from build123d import *

# Parameters (mm, degrees)
SKETCH1_W                  = 120
SKETCH1_H                  = 60
BOSS_EXTRUDE1_DEPTH        = 10
BOSS_EXTRUDE2_DEPTH        = 10
F_25_0_28_DIAMETER_HOLE1_D = 28
BOSS_EXTRUDE3_DEPTH        = 5
CUT_EXTRUDE1_DEPTH         = 147.130542204
SKETCH7_R                  = 16
SKETCH7_R_2                = 11.5
BOSS_EXTRUDE4_DEPTH        = 22.5
BOSS_EXTRUDE5_DEPTH        = 16
CUT_EXTRUDE2_START         = -10
CUT_EXTRUDE2_DEPTH         = 20
BOSS_EXTRUDE6_DEPTH        = 14.5
BOSS_EXTRUDE6_DEPTH_BACK   = 22.5
FILLET1_R                  = 2


# Read off the part's stored shape, not the designer's step: Cut-Extrude2
with BuildPart() as part:
    # Sketch1 → Boss-Extrude1 (new body)
    with BuildSketch(Plane(origin=(0, 0, 0), x_dir=(1, 0, 0), z_dir=(0, 1, 0))):
        with Locations((60, 30)):
            Rectangle(SKETCH1_W, SKETCH1_H)
    extrude(amount=BOSS_EXTRUDE1_DEPTH)

    # Sketch2 → Boss-Extrude2 (add)
    with BuildSketch(Plane.XY):
        with BuildLine():
            Line((0, 10), (0, 0))
            Line((0, 0), (70.357344256, -43.964148108))
            ThreePointArc((70.357344256, -43.964148108), (92.522919584, -46.524792309), (108.511026917, -30.960408214))
            Line((108.511026917, -30.960408214), (120, 0))
            Line((120, 0), (120, 10))
            Line((120, 10), (0, 10))
        make_face()
    boss_extrude2 = extrude(amount=-BOSS_EXTRUDE2_DEPTH)

    # Mirror1: Boss-Extrude2 across plane
    add(boss_extrude2.mirror(Plane.XY.offset(-30)))

    # 25.0 _28_ Diameter Hole1 (through all)
    with Locations(Plane(origin=(84.135245127, -21.914897608, 0), x_dir=(1, 0, 0), z_dir=(0, 0, 1))):
        with Locations((0, 0)):
            Hole(F_25_0_28_DIAMETER_HOLE1_D / 2)

    # Sketch5 → Boss-Extrude3 (add)
    with BuildSketch(Plane(origin=(0, 10, 0), x_dir=(1, 0, 0), z_dir=(0, 1, 0))):
        with BuildLine():
            Line((100, 18), (68, 18))
            ThreePointArc((68, 18), (56, 30), (68, 42))
            Line((68, 42), (100, 42))
            ThreePointArc((100, 42), (112, 30), (100, 18))
        make_face()
        with BuildLine():
            Line((100, 24), (68, 24))
            ThreePointArc((68, 24), (62, 30), (68, 36))
            Line((68, 36), (100, 36))
            ThreePointArc((100, 36), (106, 30), (100, 24))
        make_face(mode=Mode.SUBTRACT)
    extrude(amount=BOSS_EXTRUDE3_DEPTH)

    # Sketch5_2 → Cut-Extrude1 (cut, through all)
    with BuildSketch(Plane(origin=(0, 10, 0), x_dir=(1, 0, 0), z_dir=(0, 1, 0))):
        with BuildLine():
            Line((100, 36), (68, 36))
            ThreePointArc((68, 36), (62, 30), (68, 24))
            Line((68, 24), (100, 24))
            ThreePointArc((100, 24), (106, 30), (100, 36))
        make_face()
    extrude(amount=-CUT_EXTRUDE1_DEPTH, mode=Mode.SUBTRACT)



with BuildPart() as body_2:
    # Sketch7 → Boss-Extrude4 (new, symmetric)
    with BuildSketch(Plane.XY.offset(-30)):
        with Locations(Location((24.635783634, 40, 0), (0, 0, 180))):
            Circle(SKETCH7_R)
        with Locations(Location((24.635783634, 40, 0), (0, 0, 180))):
            Circle(SKETCH7_R_2, mode=Mode.SUBTRACT)
    extrude(amount=BOSS_EXTRUDE4_DEPTH, both=True)


with BuildPart() as part_1:
    add(part.part)

    add(body_2.part)  # Boss-Extrude5 merges body 2
    # Sketch7_3 → Boss-Extrude5 (add, symmetric)
    with BuildSketch(Plane.XY.offset(-30)):
        with BuildLine():
            ThreePointArc((40.635783634, 40), (35.949492133, 28.686291501), (24.635783634, 24))
            Line((24.635783634, 24), (24.635783634, 10))
            Line((24.635783634, 10), (44.852008675, 10))
            Line((44.852008675, 10), (40.635783634, 40))
        make_face()
        with BuildLine():
            ThreePointArc((24.635783634, 24), (13.322075135, 28.686291501), (8.635783634, 40))
            Line((8.635783634, 40), (4.419558593, 10))
            Line((4.419558593, 10), (24.635783634, 10))
            Line((24.635783634, 10), (24.635783634, 24))
        make_face()
    extrude(amount=BOSS_EXTRUDE5_DEPTH, both=True)

    # Cut-Extrude2 outline → Cut-Extrude2 (cut)
    with BuildSketch(Plane.XY.offset(-30).offset(CUT_EXTRUDE2_START)):
        with BuildLine():
            Line((8.635783634, 40), (4.419558593, 10))
            Line((4.419558593, 10), (44.852008675, 10))
            Line((44.852008675, 10), (40.635783634, 40))
            ThreePointArc((40.635783634, 40), (24.635783634, 24), (8.635783634, 40))
        make_face()
    extrude(amount=CUT_EXTRUDE2_DEPTH, mode=Mode.SUBTRACT)

    # Sketch7_7 → Boss-Extrude6 (add, two sides: drawn at the far end of the back side and taken through both)
    with BuildSketch(Plane.XY.offset(-30).offset(-BOSS_EXTRUDE6_DEPTH_BACK)):
        with BuildLine():
            ThreePointArc((36.135783634, 40), (32.767511617, 48.131727984), (24.635783634, 51.5))
            Line((24.635783634, 51.5), (24.635783634, 48))
            ThreePointArc((24.635783634, 48), (30.292637883, 45.656854249), (32.635783634, 40))
            ThreePointArc((32.635783634, 40), (30.292637883, 34.343145751), (24.635783634, 32))
            Line((24.635783634, 32), (24.635783634, 28.5))
            ThreePointArc((24.635783634, 28.5), (32.767511617, 31.868272016), (36.135783634, 40))
        make_face()
        with BuildLine():
            Line((24.635783634, 48), (24.635783634, 51.5))
            ThreePointArc((24.635783634, 51.5), (13.135783634, 40), (24.635783634, 28.5))
            Line((24.635783634, 28.5), (24.635783634, 32))
            ThreePointArc((24.635783634, 32), (16.635783634, 40), (24.635783634, 48))
        make_face()
    extrude(amount=BOSS_EXTRUDE6_DEPTH + BOSS_EXTRUDE6_DEPTH_BACK)

    # Fillet1
    fillet1_edges = [part_1.edges().sort_by_distance(p)[0] for p in [
        (120, 10, -30),
        (60, 10, -60),
        (114.255513458, -15.480204107, 0),
        (35.178672128, -21.982074054, 0),
        (92.522919584, -46.524792309, 0),
        (92.522919584, -46.524792309, -60),
        (114.255513458, -15.480204107, -60),
        (35.178672128, -21.982074054, -60),
        (0, 10, -30),
        (112, 10, -30),
        (84, 10, -42),
        (56, 10, -30),
        (84, 10, -18),
        (0, 5, -60),
        (120, 5, -60),
        (120, 5, 0),
        (0, 5, 0),
        (60, 10, 0),
    ]]
    fillet(fillet1_edges, radius=FILLET1_R)


solid = part_1.part
The model under review builds one solid part; all positions refer to its coordinate system, in mm. A direction names the side the tool comes from. Round coordinates to 2 decimals unless told otherwise and drop trailing zeros. Order: outer loops, then holes, each group sorted by start corner. A loop starts at its lowest first (then second) coordinate and runs counter-clockwise, first axis right, second up. Notation, with made-up numbers: (39.5, -15.75) -> (46.5, -15.75) arc R25 ccw to (46.5, 2.25) -> close; hole circle Ø1 at (16, 25). An arc over 180 degrees is marked (long way). Return JSON: item names as keys, results as strings.
1. Take a section at A-A (z = -30). Write out the cut boundary in (x, y), then the cut area to 3 significant figures.
Answer block:
{"outline": "(0, 0) -> (62, 0) -> (62, 15) -> (56, 15) -> (56, 12) arc R2 cw to (54, 10) -> (2, 10) arc R2 ccw to (0, 8) -> close; circle Ø32 at (24.64, 40); (106, 0) -> (120, 0) -> (120, 8) arc R2 ccw to (118, 10) -> (114, 10) arc R2 cw to (112, 12) -> (112, 15) -> (106, 15) -> close; hole circle Ø16 at (24.64, 40)", "area": "1,420 mm²"}
2. Insertion check: P1, Ø16, axis at x = 18.5, y = 46, coming from the -Z side; P2, Ø18.5, axis at x = 25, y = 34.5, coming from the +Z side; P3, Ø0.9, axis at x = 80, y = 14, coming from the -Z side. Each pin has a flat end and moves straight along its axis. Give the tip position at first contact, or say it passes through.
Answer block:
{"P1": "stops at z = -52.5", "P2": "stops at z = -7.5", "P3": "stops at z = -42"}
3. For L1, parallel to X at y = 40, z = -13; L2, parallel to Y at x = 31.5, z = -25.5; L3, parallel to X at y = 40, z = -27.5, list the stretches that pass through material, from the lowest coordinate up. Write a range as [from, to].
Answer block:
{"L1": "x = [8.64, 13.14], [36.14, 40.64]", "L2": "y = [0, 10], [25.55, 35.89], [44.11, 54.45]", "L3": "x = [8.64, 16.64], [32.64, 40.64]"}
4. For faces 1 (the face through (62, 8, -30)), 2 (the face through (17, 37, -52.5)), 3 (the face through (112, 13, -30)), list the 3-axis set-ups (+Z, -Z, +X, -X, +Y, -Y) from which the entire face can be reached by the end or side of a thin tool; tool diameter is ignored.
Answer block:
{"face 1": "+Y, -Y", "face 2": "-Z, +X, -X, +Y", "face 3": "+X, +Y"}
5. The part is to be moulded in two halves that separate along X. For faces 4 (the face through (0, 4, -30)), 5 (the face through (84, 8, -36)), 6 (the face through (59, 0, -30)), say which applies: +X half, -X half, draft (parallel to the pull), parting line (faces both ways), or undercut.
Answer block:
{"face 4": "-X half", "face 5": "undercut", "face 6": "draft"}
6. Take a section at B-B (y = 20). Write out the cut boundary in (x, z), then the cut area to 3 significant figures.
Answer block:
{"outline": "(5.82, -46) -> (43.45, -46) -> (43.45, -40) -> (5.82, -40) -> close; (5.82, -20) -> (43.45, -20) -> (43.45, -14) -> (5.82, -14) -> close", "area": "451 mm²"}
7. Take a section at C-C (x = 79). State how many separate pieces and enclosed holes the cut face has, then the cut area to 3 significant figures.
Answer block:
{"separate pieces": "4", "enclosed holes": "0", "area": "965 mm²"}
